Check sheet for the modelled part. Datum: model origin and axes. Units: mm. Face numbers are marked on the shaded views. A direction names the side the tool comes from. Round coordinates to 2 decimals unless told otherwise and drop trailing zeros. Write each loop counter-clockwise with the first axis right and the second up, starting at its lowest first coordinate (ties: lowest second). Pieces come first, ordered by that corner, then holes. Notation, with made-up numbers: (36.25, 15) - (43.25, 15) arc R7 cw to (43.25, 19) - close; hole circle Ø6 at (4.25, -33). An arc over 180 degrees is marked (long way). Answer as a JSON object with one key per item and string values. Group by question number.
Item 1: Thickness scan on line 1 (X direction, y = -3, z = 31); line 2 (Y direction, x = -35.5, z = 66); line 3 (Y direction, x = 57.5, z = 34). Record the ranges inside material, lowest first.
Item 2: Sectioned sample at B-B on x = 47. Record the boundary of the cut face in (y, z).
Item 3: Release check for a two-part mould opening along Y. For the marked faces 3, 4, 5 and 6 record: pulls with the +Y half, pulls with the -Y half, needs draft (parallel to the pull), parting line crosses it, or undercut.
Item 4: Set-up check for the marked faces 1 and 2: record each of +Z, -Z, +X, -X, +Y, -Y from which the full face is reachable in a straight line by a thin tool's end or side.
Item 5: Sectioned sample at C-C on x = -20.5. Record the boundary of the cut face in (y, z), plus the area to 3 significant figures.
Item 6: Gauge pin test, flat ends, axial feed: P1, Ø1.8, axis at y = 0, z = 25.5, coming from the +X side; P2, Ø1.3, axis at x = 58.5, y = 39.5, coming from the -Z side; P3, Ø2.5, axis at y = -25, z = 30, coming from the -X side; P4, Ø1.9, axis at y = 0.5, z = 20, coming from the +X side. Record the tip position at first contact, or that the pin passes through.
Item 7: Sectioned sample at A-A on y = 26. Record the boundary of the cut face in (x, z).
```python
from build123d import *

# Parameters (mm, degrees)
SKETCH_1_W          = 126
SKETCH_1_H          = 89
SKETCH_1_R          = 2.15
SKETCH_1_R_2        = 2
EXTRUDE_4_DEPTH     = 70
SKETCH_3_W          = 126
SKETCH_3_H          = 89
EXTRUDE_5_DEPTH     = 2
SKETCH_4_R          = 1.6
SKETCH_4_R_2        = 1.5
CUT_EXTRUDE_1_DEPTH = 3
SKETCH_6_R          = 1.6
CUT_EXTRUDE_3_DEPTH = 2
SKETCH_8_W          = 110
SKETCH_8_H          = 22
CUT_EXTRUDE_4_DEPTH = 8
FILLET_3_R          = 4
SKETCH_9_W          = 19
SKETCH_9_H          = 44
CUT_EXTRUDE_5_DEPTH = 2
SKETCH_10_W         = 12
SKETCH_10_H         = 2
EXTRUDE_6_DEPTH     = 22


with BuildPart() as part:
    # 草图1 → 凸台-拉伸4 (new body)
    with BuildSketch(Plane.XY):
        Rectangle(SKETCH_1_W, SKETCH_1_H)
        Polygon((-4, 42.5), (-4, 36.5), (4, 36.5), (4, 42.5), (55, 42.5), (55, 36.5), (61, 36.5), (61, -36.5), (55, -36.5), (55, -42.5), (4, -42.5), (4, -36.5), (-4, -36.5), (-4, -42.5), (-55, -42.5), (-55, -36.5), (-61, -36.5), (-61, 36.5), (-55, 36.5), (-55, 42.5), align=None, mode=Mode.SUBTRACT)
        with Locations((0, 40.5)):
            Circle(SKETCH_1_R, mode=Mode.SUBTRACT)
        with Locations((-59, 40.5)):
            Circle(SKETCH_1_R, mode=Mode.SUBTRACT)
        with Locations((0, -40.5)):
            Circle(SKETCH_1_R, mode=Mode.SUBTRACT)
        with Locations((59, -40.5)):
            Circle(SKETCH_1_R, mode=Mode.SUBTRACT)
        with Locations((59, 40.5)):
            Circle(SKETCH_1_R, mode=Mode.SUBTRACT)
        with Locations((-59, -40.5)):
            Circle(SKETCH_1_R_2, mode=Mode.SUBTRACT)
    extrude(amount=EXTRUDE_4_DEPTH)

    # 草图3 → 凸台-拉伸5 (add)
    with BuildSketch(Plane.XY.offset(70)):
        Rectangle(SKETCH_3_W, SKETCH_3_H)
    extrude(amount=EXTRUDE_5_DEPTH)

    # 草图4 → 切除-拉伸1 (cut)
    with BuildSketch(Plane(origin=(63, 0, 0), x_dir=(0, 0, -1), z_dir=(1, 0, 0))):
        with Locations((-36, 16)):
            Circle(SKETCH_4_R)
        with Locations((-4, 16)):
            Circle(SKETCH_4_R)
        with Locations((-4, -16)):
            Circle(SKETCH_4_R)
        with Locations((-36, -16)):
            Circle(SKETCH_4_R)
        with Locations((-20, 17.5)):
            Circle(SKETCH_4_R_2)
        with Locations((-20, 0)):
            Circle(SKETCH_4_R_2)
        with Locations((-20, 9.5)):
            Circle(SKETCH_4_R_2)
        with Locations((-20, 13.5)):
            Circle(SKETCH_4_R_2)
        with Locations((-20, 5.5)):
            Circle(SKETCH_4_R_2)
        with Locations((-14.592202598, 16.643489035)):
            Circle(SKETCH_4_R_2)
        with Locations((-9.713758085, 14.157797402)):
            Circle(SKETCH_4_R_2)
        with Locations((-5.842202598, 10.286241915)):
            Circle(SKETCH_4_R_2)
        with Locations((-3.356510965, 5.407797402)):
            Circle(SKETCH_4_R_2)
        with Locations((-2.5, 0)):
            Circle(SKETCH_4_R_2)
        with Locations((-3.356510965, -5.407797402)):
            Circle(SKETCH_4_R_2)
        with Locations((-5.842202598, -10.286241915)):
            Circle(SKETCH_4_R_2)
        with Locations((-9.713758085, -14.157797402)):
            Circle(SKETCH_4_R_2)
        with Locations((-14.592202598, -16.643489035)):
            Circle(SKETCH_4_R_2)
        with Locations((-20, -17.5)):
            Circle(SKETCH_4_R_2)
        with Locations((-25.407797402, -16.643489035)):
            Circle(SKETCH_4_R_2)
        with Locations((-30.286241915, -14.157797402)):
            Circle(SKETCH_4_R_2)
        with Locations((-34.157797402, -10.286241915)):
            Circle(SKETCH_4_R_2)
        with Locations((-36.643489035, -5.407797402)):
            Circle(SKETCH_4_R_2)
        with Locations((-37.5, 0)):
            Circle(SKETCH_4_R_2)
        with Locations((-36.643489035, 5.407797402)):
            Circle(SKETCH_4_R_2)
        with Locations((-34.157797402, 10.286241915)):
            Circle(SKETCH_4_R_2)
        with Locations((-30.286241915, 14.157797402)):
            Circle(SKETCH_4_R_2)
        with Locations((-25.407797402, 16.643489035)):
            Circle(SKETCH_4_R_2)
        with Locations((-14.833773663, 12.472373689)):
            Circle(SKETCH_4_R_2)
        with Locations((-10.454058454, 9.545941546)):
            Circle(SKETCH_4_R_2)
        with Locations((-7.527626311, 5.166226337)):
            Circle(SKETCH_4_R_2)
        with Locations((-6.5, 0)):
            Circle(SKETCH_4_R_2)
        with Locations((-7.527626311, -5.166226337)):
            Circle(SKETCH_4_R_2)
        with Locations((-10.454058454, -9.545941546)):
            Circle(SKETCH_4_R_2)
        with Locations((-14.833773663, -12.472373689)):
            Circle(SKETCH_4_R_2)
        with Locations((-20, -13.5)):
            Circle(SKETCH_4_R_2)
        with Locations((-25.166226337, -12.472373689)):
            Circle(SKETCH_4_R_2)
        with Locations((-29.545941546, -9.545941546)):
            Circle(SKETCH_4_R_2)
        with Locations((-32.472373689, -5.166226337)):
            Circle(SKETCH_4_R_2)
        with Locations((-33.5, 0)):
            Circle(SKETCH_4_R_2)
        with Locations((-32.472373689, 5.166226337)):
            Circle(SKETCH_4_R_2)
        with Locations((-29.545941546, 9.545941546)):
            Circle(SKETCH_4_R_2)
        with Locations((-25.166226337, 12.472373689)):
            Circle(SKETCH_4_R_2)
        with Locations((-15.25, 8.227241336)):
            Circle(SKETCH_4_R_2)
        with Locations((-11.772758664, 4.75)):
            Circle(SKETCH_4_R_2)
        with Locations((-10.5, 0)):
            Circle(SKETCH_4_R_2)
        with Locations((-11.772758664, -4.75)):
            Circle(SKETCH_4_R_2)
        with Locations((-15.25, -8.227241336)):
            Circle(SKETCH_4_R_2)
        with Locations((-20, -9.5)):
            Circle(SKETCH_4_R_2)
        with Locations((-24.75, -8.227241336)):
            Circle(SKETCH_4_R_2)
        with Locations((-28.227241336, -4.75)):
            Circle(SKETCH_4_R_2)
        with Locations((-29.5, 0)):
            Circle(SKETCH_4_R_2)
        with Locations((-28.227241336, 4.75)):
            Circle(SKETCH_4_R_2)
        with Locations((-24.75, 8.227241336)):
            Circle(SKETCH_4_R_2)
        with Locations((-16.110912703, 3.889087297)):
            Circle(SKETCH_4_R_2)
        with Locations((-14.5, 0)):
            Circle(SKETCH_4_R_2)
        with Locations((-16.110912703, -3.889087297)):
            Circle(SKETCH_4_R_2)
        with Locations((-20, -5.5)):
            Circle(SKETCH_4_R_2)
        with Locations((-23.889087297, -3.889087297)):
            Circle(SKETCH_4_R_2)
        with Locations((-25.5, 0)):
            Circle(SKETCH_4_R_2)
        with Locations((-23.889087297, 3.889087297)):
            Circle(SKETCH_4_R_2)
    extrude(amount=-CUT_EXTRUDE_1_DEPTH, mode=Mode.SUBTRACT)

    # 草图6 → 切除-拉伸3 (cut)
    with BuildSketch(Plane.ZY.offset(63)):
        with Locations((10, 34.5)):
            Circle(SKETCH_6_R)
        with Locations((20, 34.5)):
            Circle(SKETCH_6_R)
        with Locations((30, 34.5)):
            Circle(SKETCH_6_R)
        with Locations((20, 26)):
            Circle(SKETCH_6_R)
        with Locations((30, 26)):
            Circle(SKETCH_6_R)
        with Locations((20, 17.5)):
            Circle(SKETCH_6_R)
        with Locations((30, 17.5)):
            Circle(SKETCH_6_R)
        with Locations((20, 9)):
            Circle(SKETCH_6_R)
        with Locations((30, 9)):
            Circle(SKETCH_6_R)
        with Locations((20, 0.5)):
            Circle(SKETCH_6_R)
        with Locations((30, 0.5)):
            Circle(SKETCH_6_R)
        with Locations((20, -8)):
            Circle(SKETCH_6_R)
        with Locations((30, -8)):
            Circle(SKETCH_6_R)
        with Locations((20, -16.5)):
            Circle(SKETCH_6_R)
        with Locations((30, -16.5)):
            Circle(SKETCH_6_R)
        with Locations((20, -25)):
            Circle(SKETCH_6_R)
        with Locations((30, -25)):
            Circle(SKETCH_6_R)
        with Locations((20, -33.5)):
            Circle(SKETCH_6_R)
        with Locations((30, -33.5)):
            Circle(SKETCH_6_R)
        with Locations((10, 26)):
            Circle(SKETCH_6_R)
        with Locations((10, 17.5)):
            Circle(SKETCH_6_R)
        with Locations((10, 9)):
            Circle(SKETCH_6_R)
        with Locations((10, 0.5)):
            Circle(SKETCH_6_R)
        with Locations((10, -8)):
            Circle(SKETCH_6_R)
        with Locations((10, -16.5)):
            Circle(SKETCH_6_R)
        with Locations((10, -25)):
            Circle(SKETCH_6_R)
        with Locations((10, -33.5)):
            Circle(SKETCH_6_R)
    extrude(amount=-CUT_EXTRUDE_3_DEPTH, mode=Mode.SUBTRACT)

    # 草图8 → 切除-拉伸4 (cut)
    with BuildSketch(Plane.XZ.offset(44.5)):
        with Locations((0, 11)):
            Rectangle(SKETCH_8_W, SKETCH_8_H)
    extrude(amount=-CUT_EXTRUDE_4_DEPTH, mode=Mode.SUBTRACT)

    # 圆角3
    fillet_3_edges = [part.edges().sort_by_distance(p)[0] for p in [
        (-55, 36.5, 35),
        (-55, -36.5, 35),
        (-63, 44.5, 36),
        (-63, -44.5, 36),
        (4, -36.5, 46),
        (-4, -36.5, 46),
        (4, 36.5, 35),
        (-4, 36.5, 35),
        (55, -36.5, 35),
        (63, -44.5, 36),
        (63, 44.5, 36),
        (55, 36.5, 35),
    ]]
    fillet(fillet_3_edges, radius=FILLET_3_R - 0.0001)  # a hair under: the kernel refuses the full size

    # 草图9 → 切除-拉伸5 (cut)
    with BuildSketch(Plane.ZY.offset(-61)):
        with Locations((57.5, 1.907407407)):
            Rectangle(SKETCH_9_W, SKETCH_9_H)
    extrude(amount=-CUT_EXTRUDE_5_DEPTH, mode=Mode.SUBTRACT)

    # 草图10 → 凸台-拉伸6 (add)
    with BuildSketch(Plane(origin=(0, 0, 22), x_dir=(-1, 0, 0), z_dir=(0, 0, -1))):
        with Locations((-49, -43.5)):
            Rectangle(SKETCH_10_W, SKETCH_10_H)
    extrude(amount=EXTRUDE_6_DEPTH)


solid = part.part
```
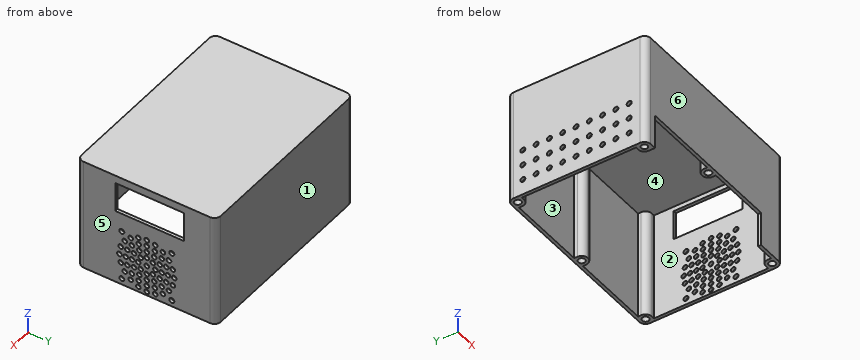
Completed:
{
 "1": {"line 1": "-63 to -61, 61 to 63", "line 2": "-44.5 to -42.5, 42.5 to 44.5", "line 3": "-44.5 to -42.04, -38.96 to -36.79, 36.79 to 38.96, 42.04 to 44.5"},
 "2": {"outline": "(-44.5, 0) - (-42.5, 0) - (-42.5, 70) - (42.5, 70) - (42.5, 0) - (44.5, 0) - (44.5, 72) - (-44.5, 72) - close"},
 "3": {"face 3": "undercut", "face 4": "undercut", "face 5": "needs draft", "face 6": "pulls with the -Y half"},
 "4": {"face 1": "+Z, -Z, +X, -X, +Y", "face 2": "-Z"},
 "5": {"outline": "(-44.5, 22) - (-42.5, 22) - (-42.5, 70) - (42.5, 70) - (42.5, 0) - (44.5, 0) - (44.5, 72) - (-44.5, 72) - close", "area": "414 mm²"},
 "6": {"P1": "x = -61", "P2": "z = 70", "P3": "x = 61", "P4": "through"},
 "7": {"outline": "(-63, 0) - (-61, 0) - (-61, 8.4) - (-63, 8.4) - close; (-63, 11.6) - (-61, 11.6) - (-61, 18.4) - (-63, 18.4) - close; (-63, 21.6) - (-61, 21.6) - (-61, 28.4) - (-63, 28.4) - close; (-63, 31.6) - (-61, 31.6) - (-61, 70) - (61, 70) - (61, 0) - (63, 0) - (63, 72) - (-63, 72) - close"}
}
